Verification items for the finished model (mm, model axes). A direction names the side the tool comes from. Give positions to 0.01 mm unless a question says otherwise; leave off trailing zeros. Loops run counter-clockwise (first coordinate to the right, second up) from the corner with the lowest first, then second, coordinate; pieces in that order, holes last. Notation, with made-up numbers: (89.5, 38.25) - (100.5, 38.25) arc R17 ccw to (100.5, 49.25) - close; hole circle Ø9 at (77, -15). An arc over 180 degrees is marked (long way). One line per item, written item: value. Start each with the question number.
1. Sectioned sample at A-A (z = -17.5). Record the cut outline in (x, y), plus the area to 3 significant figures.
2. Sectioned sample at B-B (x = 90.2). Record the cut outline in (y, z).
3. Access from +Z, -Z, +X, -X, +Y, -Y to the whole of each face (thin tool, end or side, straight path). Record for faces 5 (the flat face through (54, 2, -28)), 6 (the flat face through (29, 1, -45)), 7 (the flat face through (55, -26, -1)), 8 (the cylindrical face through (71.481, -0.855, -1.232)), 9 (the flat face through (54, -16, -2.5)).
4. Sectioned sample at C-C (y = -6). Record the cut outline in (x, z), plus the area to 3 significant figures.
5. Scan lines: L1, parallel to X at y = 0.5, z = -38; L2, parallel to Z at x = 90.2, y = 1.1; L3, parallel to Y at x = 103, z = -40. Record each from-to range of solid material in increasing order. Write a range as [from, to].
6. Mould release check, pull along X, two halves, no side actions. Record for faces 1 (the cylindrical face through (10.193, 0.986, -43.496)), 2 (the flat face through (54, -15, 0)), 3 (the flat face through (55, -13, -1)), 4 (the flat face through (0, 1, -28)): pulls with the +X half, pulls with the -X half, needs draft (parallel to the pull), parting line crosses it, or undercut.
7. Gauge pin test, flat ends, axial feed: pin 1 (1 mm diameter, centred on x = 92.5, z = -7, fed in from -Y); pin 2 (1.2 mm diameter, centred on y = -12.5, z = -1, fed in from -X); pin 3 (2.5 mm diameter, centred on x = 90.2, z = -50.7, fed in from -Y); pin 4 (1.2 mm diameter, centred on y = -9.5, z = -2, fed in from +X). Record the tip position at first contact, or that the pin passes through.
8. Sectioned sample at D-D (x = 77). Record the cut outline in (y, z), plus the area to 3 significant figures.
from build123d import *

# Parameters (mm, degrees)
SKETCH_1_R          = 1.7
EXTRUDE_2_DEPTH     = 2
SKETCH_2_W          = 65
SKETCH_2_H          = 2.5
EXTRUDE_3_DEPTH     = 30
SKETCH_3_R          = 2.25
CUT_EXTRUDE_1_DEPTH = 2.5


with BuildPart() as part:
    # 草图1 → 凸台-拉伸2 (new body)
    with BuildSketch(Plane(origin=(0, 0, 0), x_dir=(1, 0, 0), z_dir=(0, 1, 0))):
        with BuildLine():
            Line((5, 0), (105, 0))
            ThreePointArc((105, 0), (108.535533906, 1.464466094), (110, 5))
            Line((110, 5), (110, 50))
            ThreePointArc((110, 50), (108.535533906, 53.535533906), (105, 55))
            Line((105, 55), (5, 55))
            ThreePointArc((5, 55), (1.464466094, 53.535533906), (0, 50))
            Line((0, 50), (0, 5))
            ThreePointArc((0, 5), (1.464466094, 1.464466094), (5, 0))
        make_face()
        with Locations(Location((14, 2.5, 0), (0, 0, 270))):
            Circle(SKETCH_1_R, mode=Mode.SUBTRACT)
        with Locations(Location((15.3, 50.7, 0), (0, 0, 270))):
            Circle(SKETCH_1_R, mode=Mode.SUBTRACT)
        with Locations(Location((90.2, 50.7, 0), (0, 0, 270))):
            Circle(SKETCH_1_R, mode=Mode.SUBTRACT)
        with Locations(Location((96.6, 2.5, 0), (0, 0, 270))):
            Circle(SKETCH_1_R, mode=Mode.SUBTRACT)
        with BuildLine():
            Line((13.766884745, 45), (43.750231267, 45))
            ThreePointArc((43.750231267, 45), (47.285765173, 43.535533906), (48.750231267, 40))
            Line((48.750231267, 40), (48.750231267, 14))
            ThreePointArc((48.750231267, 14), (47.285765173, 10.464466094), (43.750231267, 9))
            Line((43.750231267, 9), (13.766884745, 9))
            ThreePointArc((13.766884745, 9), (10.231350839, 10.464466094), (8.766884745, 14))
            Line((8.766884745, 14), (8.766884745, 40))
            ThreePointArc((8.766884745, 40), (10.231350839, 43.535533906), (13.766884745, 45))
        make_face(mode=Mode.SUBTRACT)
        with BuildLine():
            Line((66.201792467, 45), (94.663281509, 45))
            ThreePointArc((94.663281509, 45), (98.198815415, 43.535533906), (99.663281509, 40))
            Line((99.663281509, 40), (99.663281509, 14))
            ThreePointArc((99.663281509, 14), (98.198815415, 10.464466094), (94.663281509, 9))
            Line((94.663281509, 9), (66.201792467, 9))
            ThreePointArc((66.201792467, 9), (62.666258562, 10.464466094), (61.201792467, 14))
            Line((61.201792467, 14), (61.201792467, 40))
            ThreePointArc((61.201792467, 40), (62.666258562, 43.535533906), (66.201792467, 45))
        make_face(mode=Mode.SUBTRACT)
    extrude(amount=EXTRUDE_2_DEPTH)

    # 草图2 → 凸台-拉伸3 (add)
    with BuildSketch(Plane.XZ):
        with Locations((54.883282113, -1.25)):
            Rectangle(SKETCH_2_W, SKETCH_2_H)
    extrude(amount=EXTRUDE_3_DEPTH)

    # 草图3 → 切除-拉伸1 (cut)
    with BuildSketch(Plane.XY):
        with Locations((77.383282113, -18)):
            Circle(SKETCH_3_R)
        with Locations((32.383282113, -18)):
            Circle(SKETCH_3_R)
        Polygon((87.383282113, -30), (87.383282113, -23), (82.383282113, -26), (27.383282113, -26), (22.383282113, -23), (22.383282113, -30), align=None)
        with BuildLine():
            Line((69.383282113, -13), (40.383282113, -13))
            ThreePointArc((40.383282113, -13), (38.26196177, -12.121320344), (37.383282113, -10))
            Line((37.383282113, -10), (37.383282113, -3))
            ThreePointArc((37.383282113, -3), (38.26196177, -0.878679656), (40.383282113, 0))
            Line((40.383282113, 0), (69.383282113, 0))
            ThreePointArc((69.383282113, 0), (71.504602457, -0.878679656), (72.383282113, -3))
            Line((72.383282113, -3), (72.383282113, -10))
            ThreePointArc((72.383282113, -10), (71.504602457, -12.121320344), (69.383282113, -13))
        make_face()
    extrude(amount=-CUT_EXTRUDE_1_DEPTH, mode=Mode.SUBTRACT)


solid = part.part
Results are:
1. outline: (0, 0) - (8.77, 0) - (8.77, 2) - (0, 2) - close; (48.75, 0) - (61.2, 0) - (61.2, 2) - (48.75, 2) - close; (99.66, 0) - (110, 0) - (110, 2) - (99.66, 2) - close
1. area: 63.1 mm^2
2. outline: (0, -55) - (2, -55) - (2, -52.4) - (0, -52.4) - close; (0, -49) - (2, -49) - (2, -45) - (0, -45) - close; (0, -9) - (2, -9) - (2, 0) - (0, 0) - close
3. face 5: +Z, -Z, +X, -X, +Y
3. face 6: +Y, -Y
3. face 7: +Z, -Z, +X, -X, -Y
3. face 8: +Z, -Z
3. face 9: -Z, +X, -X, -Y
4. outline: (22.38, -2.5) - (37.38, -2.5) - (37.38, 0) - (22.38, 0) - close; (72.38, -2.5) - (87.38, -2.5) - (87.38, 0) - (72.38, 0) - close
4. area: 75.0 mm^2
5. L1: x = [0, 8.77], [48.75, 61.2], [99.66, 110]
5. L2: z = [-55, -52.4], [-49, -45], [-9, 0]
5. L3: y = [0, 2]
6. face 1: undercut
6. face 2: needs draft
6. face 3: undercut
6. face 4: pulls with the -X half
7. pin 1: stops at y = 0
7. pin 2: stops at x = 22.38
7. pin 3: passes through
7. pin 4: stops at x = 87.38
8. outline: (-26, -2.5) - (-20.22, -2.5) - (-20.22, 0) - (-26, 0) - close; (-15.78, -2.5) - (0, -2.5) - (0, -9) - (2, -9) - (2, 0) - (-15.78, 0) - close; (0, -55) - (2, -55) - (2, -45) - (0, -45) - close
8. area: 91.9 mm^2
